For this review, take the finished solid that the model builds, in its own axes (mm). Coordinates: 2 decimals unless noted, no trailing zeros. Loops run counter-clockwise (first coordinate to the right, second up) from the corner with the lowest first, then second, coordinate; pieces in that order, holes last. Notation, with made-up numbers: (0, 52.5) -> (52, 52.5) arc R23 cw to (52, 91.5) -> close; hole circle Ø4 at (18, 7). An arc over 180 degrees is marked (long way). Answer in a Markdown table with one row per item.
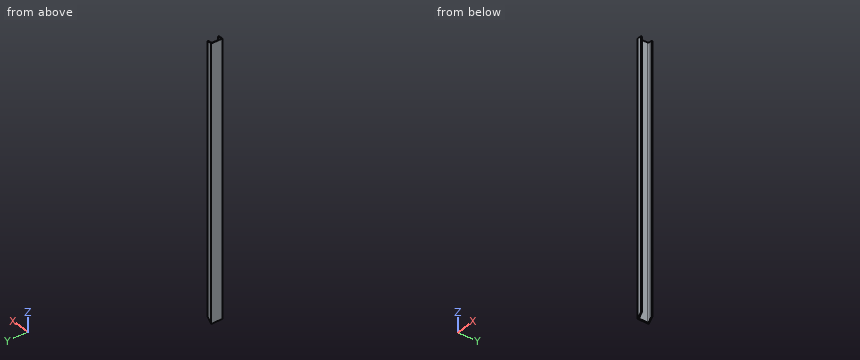
Autodesk Inventor part; units mm, degrees
ref_plane "Start plane" through (0, 0, 0) normal (0, 0, 1) x (1, 0, 0)
ref_plane "End plane" through (0, 0, 2438.4) normal (0, 0, 1) x (1, 0, 0)
ref_plane "Work Plane4" through (0, 0, 0) normal (0.7071, 0, -0.7071) x (-0.7071, 0, -0.7071)
ref_plane "Start plane" through (0, 0, 0) normal (0, 0, 1) x (1, 0, 0)
ref_plane "End plane" through (0, 0, 2438.4) normal (0, 0, 1) x (1, 0, 0)
sketch "Sketch" plane through (0, 0, 0) normal (0, 0, 1) x (1, 0, 0)
  line L0 (0, 0) -> (0, 50.8)
  line L1 (0, 50.8) -> (40.2336, 50.8)
  line L2 (40.2336, 50.8) -> (40.2336, 46.3293)
  line L3 (38.1154, 44.0972) -> (11.035, 42.6782)
  line L4 (4.6736, 35.9747) -> (4.6736, 0)
  line L5 (4.6736, 0) -> (0, 0) construction
  line L6 (22.5508, 50.8) -> (22.5508, 43.2816) construction
  line L7 (40.2336, 44.2082) -> (40.2336, 43.2816) construction
  line L8 (40.2336, 43.2816) -> (22.5508, 43.2816) construction
  line L9 (0, 15) -> (0, -27) construction
  line L10 (-5.539, 0) -> (16.0067, 0) construction
  line L11 (0, 0) -> (0, -50.8)
  line L12 (0, -50.8) -> (40.2336, -50.8)
  line L13 (40.2336, -50.8) -> (40.2336, -46.3293)
  line L14 (38.1154, -44.0972) -> (11.035, -42.6782)
  line L15 (4.6736, -35.9747) -> (4.6736, 0)
  arc A0 (11.035, 42.6782) -> (4.6736, 35.9747) centre (11.3862, 35.9747) ccw
  arc A1 (4.6736, -35.9747) -> (11.035, -42.6782) centre (11.3862, -35.9747) ccw
  arc A2 (38.1154, 44.0972) -> (40.2336, 46.3293) centre (37.9984, 46.3293) ccw
  arc A3 (40.2336, -46.3293) -> (38.1154, -44.0972) centre (37.9984, -46.3293) ccw
  line L16 (0, 71.12) -> (0, -71.12) construction
  line L17 (-14.7825, 0) -> (49.9224, 0) construction
  point P0 (4.6736, 42.3448)
  point P1 (40.2336, -44.2082)
  point P2 (4.6736, -42.3448)
  point P3 (22.5508, -50.8)
  point P4 (22.5508, -43.2816)
  dimension "d0" = 4.6736
  dimension "d1" = 50.8
  dimension "d2" = 40.2336
  dimension "d3" = 7.5184
  dimension "d4" = 17.6828
  dimension "d5" = 0.9266
  dimension "d25" = 0
  dimension "d28" = 6.7127
  dimension "d29" = 2.2352
extrude "Body" add sketch "Sketch" along normal up to surface (2438.4 mm away) from surface at 0
sketch "Sketch3" plane through (0, 0, 0) normal (0, 0, 1) x (1, 0, 0)
  line L0 (0, 0) -> (10, 0)
ref_plane "Work Plane3" through (0, 0, 0) normal (0, -1, 0) x (1, 0, 0)
sketch "Sketch4" plane through (0, 0, 0) normal (0, -1, 0) x (1, 0, 0)
  line L0 (-2, 0) -> (12, 0)
  line L1 (-2, 2438.4) -> (12, 2438.4)
  dimension "d31" = 2438.4
ref_plane "Work Plane4" through (0, 0, 0) normal (0.7071, 0, -0.7071) x (-0.7071, 0, -0.7071)
split "Split1" plane through (0, 0, 0) removes the side toward (0.7071, 0, -0.7071)
equation "\"d0\" = G_T"
equation "\"d1\" = 0.5 * G_H"
equation "\"d2\" = G_W"
equation "\"d3\" = G_T1"
equation "\"d4\" = G_C"
equation "\"d28\" = G_IR"
equation "\"d29\" = G_ER"
equation "\"d6\" = G_L"
equation "\"G_W\" = 40.2336"
equation "\"G_H\" = 101.6"
equation "\"G_T\" = 4.6736"
equation "\"G_T1\" = 7.5184"
equation "\"G_NG\" = 0.0524"
equation "\"G_ER\" = 2.2352"
equation "\"G_IR\" = 6.71265"
equation "\"G_C\" = 17.68285"
equation "\"G_L\" = d31"
equation "\"ex\" = 0"
equation "\"G_OFFSET_START\" = 0"
equation "\"G_OFFSET_END\" = 0"
equation "\"d27\" = G_OFFSET_END + B_L"
equation "\"B_L\" = 2438.4"
properties part number "AISC - C 4 x 5.4 - 96" material "Steel, Mild"
Item 1: Take a section at A-A, the plane x = 21. State the section outline as (y, z) points.
Worked answers:
| item | result |
|---|---|
| outline | (-50.8, 21) -> (-43.2, 21) -> (-43.2, 2438.4) -> (-50.8, 2438.4) -> close; (43.2, 21) -> (50.8, 21) -> (50.8, 2438.4) -> (43.2, 2438.4) -> close |
Item 2: Take a section at B-B, the plane z = 2289.5. State the section outline as (x, y) points (3 decimals), and give its area (3 significant figures).
Worked answers:
| item | result |
|---|---|
| outline | (0, -50.8) -> (40.234, -50.8) -> (40.234, -46.329) arc R2.235 ccw to (38.115, -44.097) -> (11.035, -42.678) arc R6.713 cw to (4.674, -35.975) -> (4.674, 35.975) arc R6.713 cw to (11.035, 42.678) -> (38.115, 44.097) arc R2.235 ccw to (40.234, 46.329) -> (40.234, 50.8) -> (0, 50.8) -> close |
| area | 1,030 mm² |
Item 3: For L1, parallel to Y at x = 19, z = 182; L2, parallel to Y at x = 36, z = 2091.5; L3, parallel to X at y = 34.5, z = 989, list the stretches that pass through material, from the lowest coordinate up.
Worked answers:
| item | result |
|---|---|
| L1 | -50.8 to -43.1, 43.1 to 50.8 |
| L2 | -50.8 to -43.99, 43.99 to 50.8 |
| L3 | 0 to 4.67 |
Item 4: Take a section at C-C, the plane y = 1.5. State the section outline as (x, z) points.
Worked answers:
| item | result |
|---|---|
| outline | (0, 0) -> (4.67, 4.67) -> (4.67, 2438.4) -> (0, 2438.4) -> close |
Item 5: Insertion check: pin 1 (5 mm diameter, centred on y = -34, z = 423.5, fed in from +X). The pin has a flat end and moves straight along its axis. Give the tip position at first contact, or say it passes through.
Worked answers:
| item | result |
|---|---|
| pin 1 | x = 4.69 |
